from build123d import *

# Parameters (mm, degrees)
SKETCH2_W                                           = 90.17
SKETCH2_H                                           = 22.098
BOSS_EXTRUDE1_DEPTH                                 = 17.78
SKETCH3_W                                           = 66.04
SKETCH3_H                                           = 2.54
BOSS_EXTRUDE2_DEPTH                                 = 12.7
CBORE_FOR_8_BINDING_HEAD_MACHINE_SCREW1_D           = 3.81
CBORE_FOR_8_BINDING_HEAD_MACHINE_SCREW1_CBORE_D     = 7.62
CBORE_FOR_8_BINDING_HEAD_MACHINE_SCREW1_CBORE_DEPTH = 11.176


with BuildPart() as part:
    # Sketch2 → Boss-Extrude1 (new body)
    with BuildSketch(Plane(origin=(0, 0, 0), x_dir=(1, 0, 0), z_dir=(0, 1, 0))):
        with Locations((45.085, 11.049)):
            Rectangle(SKETCH2_W, SKETCH2_H)
    extrude(amount=BOSS_EXTRUDE1_DEPTH)

    # Sketch3 → Boss-Extrude2 (add)
    with BuildSketch(Plane.XY):
        with Locations((45.085, 11.117631295)):
            Rectangle(SKETCH3_W, SKETCH3_H)
    extrude(amount=BOSS_EXTRUDE2_DEPTH)

    # CBORE for #8 Binding Head Machine Screw1 (through all)
    with Locations(Plane(origin=(0, 17.78, 0), x_dir=(1, 0, 0), z_dir=(0, 1, 0))):
        with Locations((5.3975, 10.814852879), (84.7725, 10.814852879)):
            CounterBoreHole(CBORE_FOR_8_BINDING_HEAD_MACHINE_SCREW1_D / 2, CBORE_FOR_8_BINDING_HEAD_MACHINE_SCREW1_CBORE_D / 2, CBORE_FOR_8_BINDING_HEAD_MACHINE_SCREW1_CBORE_DEPTH)


solid = part.part
Design review of the part built by this model. Coordinates are the model's own, in mm. A direction names the side the tool comes from. Round coordinates to 2 decimals unless told otherwise and drop trailing zeros. Write each loop counter-clockwise with the first axis right and the second up, starting at its lowest first coordinate (ties: lowest second). Pieces come first, ordered by that corner, then holes. Notation, with made-up numbers: M 29,20.25 L 87,20.25 A18 cw 87,27.25 Z; hole C 86,-13 d5. An arc over 180 degrees is marked long. One line per item, written item: value. Start each with the question number.
1. Clearance check with flat-ended pins moving along their axes: P1, Ø3, axis at x = 5.4, z = -10.81, coming from the -Y side; P2, Ø8, axis at y = 7, z = 5, coming from the +X side (3 decimals); P3, Ø4, axis at x = 84, z = -10, coming from the +Y side; P4, Ø3, axis at y = 11.5, z = 4.5, coming from the -X side (3 decimals). State where each tip first meets the part, or that it passes through.
2. To check wall thickness, follow probe 1 along Y at (x, z) = (44, 4); probe 2 along Z at (x, y) = (6.5, 11.5); probe 3 along X at (y, z) = (11.25, 1) (3 decimals). State the ranges of each line that lie inside material, in increasing order. Write a range as from..to.
3. Take a section at D-D on z = 1. State the section outline as (x, y) points (3 decimals), then the cut area to 3 significant figures.
4. Take a section at C-C on y = 15.5. State the section outline as (x, z) points, then the cut area to 3 significant figures.
5. Draft analysis for pull direction Z (two halves, no side actions). For faces 1 (the face through (6, 6.604, -13)), 2 (the face through (90.17, 9, -11)), 3 (the face through (44, 9, -22.098)), 4 (the face through (80.966, 12.27, -10.982)), state which applies: pulls with the +Z half, pulls with the -Z half, needs draft (parallel to the pull), parting line crosses it, or undercut.
6. Take a section at A-A on x = 85. State the section outline as (y, z) points, then the cut area to 3 significant figures.
7. For faces 5 (the face through (45, 12.388, 6)), 6 (the face through (12.065, 11, 6)), 7 (the face through (86, 6.604, -13)), list the 3-axis set-ups (+Z, -Z, +X, -X, +Y, -Y) from which the entire face can be reached by the end or side of a thin tool; tool diameter is ignored.
8. Take a section at B-B on x = 42. State the section outline as (y, z) points.
Computed:
1. P1: passes through
1. P2: stops at x = 78.105
1. P3: stops at y = 6.6
1. P4: stops at x = 12.065
2. probe 1: y = 9.85..12.39
2. probe 2: z = -22.1..-14.46, -7.17..0
2. probe 3: x = 12.065..78.105
3. outline: M 12.065,9.848 L 78.105,9.848 L 78.105,12.388 L 12.065,12.388 Z
3. area: 168 mm²
4. outline: M 0,-22.1 L 90.17,-22.1 L 90.17,0 L 0,0 Z; hole C 5.4,-10.81 d7.62; hole C 84.77,-10.81 d7.62
4. area: 1,900 mm²
5. face 1: undercut
5. face 2: needs draft
5. face 3: pulls with the -Z half
5. face 4: undercut
6. outline: M 0,-22.1 L 17.78,-22.1 L 17.78,-14.62 L 6.6,-14.62 L 6.6,-12.71 L 0,-12.71 Z; M 0,-8.92 L 6.6,-8.92 L 6.6,-7.01 L 17.78,-7.01 L 17.78,0 L 0,0 Z
6. area: 283 mm²
7. face 5: +Z, +X, -X, +Y
7. face 6: +Z, -X, +Y, -Y
7. face 7: +Y
8. outline: M 0,-22.1 L 17.78,-22.1 L 17.78,0 L 12.39,0 L 12.39,12.7 L 9.85,12.7 L 9.85,0 L 0,0 Z
